Work out the finished part from the listing and answer in its coordinate system (mm). A direction names the side the tool comes from. Coordinates: 2 decimals unless noted, no trailing zeros. Write each loop counter-clockwise with the first axis right and the second up, starting at its lowest first coordinate (ties: lowest second). Pieces come first, ordered by that corner, then holes. Notation, with made-up numbers: (39.5, 72) - (91.5, 72) arc R13 ccw to (91.5, 83) - close; hole circle Ø8 at (54.5, 7). An arc over 180 degrees is marked (long way). Use one line per item in the form item = value. Start each with the question number.
Item 1: Consider probe 1 along X at (y, z) = (12, -0.2); probe 2 along Y at (x, z) = (57.5, 0.2); probe 3 along Y at (x, z) = (53.5, 0). Determine where each line is inside the solid, lowest interval first.
Item 2: A cutting plane is placed at A-A (x = -4). Write down the section's boundary in (y, z), then the cut area to 3 significant figures.
Item 3: Determine the mould class of faces 1 (the flat face through (-1, 0, -0.8)), 2 (the cylindrical face through (-36.546, 12.3, -0.011)), 3 (the cylindrical face through (3.263, -6.324, -0.011)) for opening direction Y: released by +Y, released by -Y, zero draft, split by the parting line, or undercut.
Item 4: A cutting plane is placed at C-C (z = -0.05). Give the number of separate pieces and of enclosed holes in the cut face, then the cut area to 3 significant figures.
Item 5: A cutting plane is placed at B-B (x = -24). Write down the section's boundary in (y, z), then the cut area to 3 significant figures.
Item 6: Given pin 1 (1.8 mm diameter, centred on x = 4, y = -7, fed in from +Z), flat-ended and moving along its own axis, determine where the tip first touches the part or whether it passes through.
Item 7: For faces 4 (the flat face through (-1, 0, 0.8)), 5 (the flat face through (-23.9, -5.5, 0)), determine the directions among +Z, -Z, +X, -X, +Y, -Y from which every point of the face is accessible in a straight line to the end or side of a thin tool.
from build123d import *

# Parameters (mm, degrees)
SKETCH1_W               = 120
SKETCH1_H               = 34.5
BOSS_EXTRUDE1_DEPTH     = 0.8
CUT_EXTRUDE1_DEPTH      = 65.82908298
CUT_EXTRUDE1_DEPTH_BACK = 65.82908298
SKETCH2_R               = 1
SKETCH2_R_2             = 0.75
FILLET1_R               = 0.5


with BuildPart() as part:
    # Sketch1 → Boss-Extrude1 (new, symmetric)
    with BuildSketch(Plane.XY):
        with Locations((0, 7.25)):
            Rectangle(SKETCH1_W, SKETCH1_H)
    extrude(amount=BOSS_EXTRUDE1_DEPTH, both=True)

    # Sketch2 → Cut-Extrude1 (cut, two sides: drawn at the far end of the back side and taken through both)
    with BuildSketch(Plane.XY.offset(0.8).offset(-CUT_EXTRUDE1_DEPTH_BACK)):
        with Locations((-37.5, 12)):
            Circle(SKETCH2_R)
        with Locations((-4, -7)):
            Circle(SKETCH2_R)
        with Locations((37.5, 12)):
            Circle(SKETCH2_R)
        with Locations((-57.5, 1.25)):
            Circle(SKETCH2_R)
        with Locations(Location((57.5, 1.25, 0), (0, 0, 180))):
            Circle(SKETCH2_R)
        with Locations((4, -7)):
            Circle(SKETCH2_R)
        with Locations((-18.005, 22)):
            Circle(SKETCH2_R)
        with Locations(Location((18.005, 22, 0), (0, 0, 180))):
            Circle(SKETCH2_R)
        with Locations((37.618090351, 17.2224)):
            Circle(SKETCH2_R_2)
        with Locations(Location((-37.618090351, 17.2224, 0), (0, 0, 180))):
            Circle(SKETCH2_R_2)
        with BuildLine():
            Line((-26.4, -8), (-58.4, -8))
            Line((-58.4, -8), (-58.4, -1.25))
            Line((-58.4, -1.25), (-57.5, -1.25))
            ThreePointArc((-57.5, -1.25), (-55.732233047, -0.517766953), (-55, 1.25))
            Line((-55, 1.25), (-55, 4))
            Line((-55, 4), (-26.4, 4))
            Line((-26.4, 4), (-21.4, 4))
            Line((-21.4, 4), (-21.4, -3))
            Line((-21.4, -3), (-26.4, -8))
        make_face()
        Polygon((-58.4, 22.9), (-38.9, 22.9), (-38.9, 21.4), (-47.4, 12.9), (-58.4, 12.9), align=None)
        Polygon((7.746, 24.5), (-7.746, 24.5), (-7.746, 3.5), (-5.756, 1.51), (5.756, 1.51), (7.746, 3.5), align=None)
        Polygon((58.4, 22.9), (58.4, 12.9), (47.4, 12.9), (38.9, 21.4), (38.9, 22.9), align=None)
        with BuildLine():
            Line((21.4, 4), (21.4, -3))
            Line((21.4, -3), (26.4, -8))
            Line((26.4, -8), (58.4, -8))
            Line((58.4, -8), (58.4, -1.25))
            Line((58.4, -1.25), (57.5, -1.25))
            ThreePointArc((57.5, -1.25), (55.732233047, -0.517766953), (55, 1.25))
            Line((55, 1.25), (55, 4))
            Line((55, 4), (26.4, 4))
            Line((26.4, 4), (21.4, 4))
        make_face()
    extrude(amount=CUT_EXTRUDE1_DEPTH + CUT_EXTRUDE1_DEPTH_BACK, mode=Mode.SUBTRACT)

    # Fillet1
    fillet1_edges = [part.edges().sort_by_distance(p)[0] for p in [
        (-7.746, 3.5, 0),
        (-5.756, 1.51, 0),
        (5.756, 1.51, 0),
        (7.746, 3.5, 0),
        (-26.4, -8, 0),
        (-58.4, -8, 0),
        (-21.4, -3, 0),
        (-21.4, 4, 0),
        (-55, 4, 0),
        (-58.4, -1.25, 0),
        (21.4, -3, 0),
        (26.4, -8, 0),
        (58.4, -8, 0),
        (58.4, -1.25, 0),
        (55, 4, 0),
        (21.4, 4, 0),
        (-58.4, 22.9, 0),
        (-38.9, 22.9, 0),
        (-58.4, 12.9, 0),
        (-47.4, 12.9, 0),
        (-38.9, 21.4, 0),
        (58.4, 22.9, 0),
        (58.4, 12.9, 0),
        (38.9, 22.9, 0),
        (38.9, 21.4, 0),
        (47.4, 12.9, 0),
    ]]
    fillet(fillet1_edges, radius=FILLET1_R)


solid = part.part
Answer:
q1.probe_1 = -60 to -38.5, -36.5 to -7.75, 7.75 to 36.5, 38.5 to 60
q1.probe_2 = -10 to -8, -1.25 to 0.25, 2.25 to 12.9, 22.9 to 24.5
q1.probe_3 = -10 to -8, 4 to 12.9, 22.9 to 24.5
q2.outline = (-10, -0.8) - (-8, -0.8) - (-8, 0.8) - (-10, 0.8) - close; (-6, -0.8) - (1.51, -0.8) - (1.51, 0.8) - (-6, 0.8) - close
q2.area = 15.2 mm²
q3.face_1 = zero draft
q3.face_2 = undercut
q3.face_3 = undercut
q4.separate_pieces = 1
q4.enclosed_holes = 14
q4.area = 2,610 mm²
q5.outline = (-10, -0.8) - (-5.6, -0.8) - (-5.6, 0.8) - (-10, 0.8) - close; (4, -0.8) - (24.5, -0.8) - (24.5, 0.8) - (4, 0.8) - close
q5.area = 39.8 mm²
q6.pin_1 = through
q7.face_4 = +Z, +X, -X, +Y, -Y
q7.face_5 = +Z, -Z
